Verification items for the finished model (mm, model axes). Face numbers are marked on the shaded views. A direction names the side the tool comes from. Coordinates: 2 decimals unless noted, no trailing zeros. Loops run counter-clockwise (first coordinate to the right, second up) from the corner with the lowest first, then second, coordinate; pieces in that order, holes last. Notation, with made-up numbers: (-24, 17.25) - (-13, 17.25) arc R21 cw to (-13, 44.25) - close; hole circle Ø1 at (88, 42). An arc over 180 degrees is marked (long way). One line per item, written item: value. Start each with the question number.
(1) Draft check along X on the marked faces 6, 7 and 8. Enter one of: +X half, -X half, draft (parallel to the pull), parting line (faces both ways), or undercut.
(2) Set-up check for the marked faces 1, 2, 3, 4 and 5: record each of +Z, -Z, +X, -X, +Y, -Y from which the full face is reachable in a straight line by a thin tool's end or side.
(3) Section check A-A (x = 99). Record the boundary of the cut face in (y, z).
(4) Section check C-C (x = 104). Record the boundary of the cut face in (y, z), plus the area to 3 significant figures.
(5) Gauge pin test, flat ends, axial feed: P1, Ø0.5, axis at y = -1, z = 0.5, coming from the -X side; P2, Ø0.5, axis at x = 108, z = 0.5, coming from the +Y side; P3, Ø2, axis at x = 101, y = -4.5, coming from the -Z side; P4, Ø0.8, axis at y = -0.5, z = 0.5, coming from the +X side. Record the tip position at first contact, or that the pin passes through.
(6) Section check B-B (x = 112.25). Record the boundary of the cut face in (y, z).
(7) Thickness scan on probe 1 along X at (y, z) = (-1, 0.9); probe 2 along X at (y, z) = (-0.75, 1.45); probe 3 along X at (y, z) = (3.25, 1.35). Record the ranges inside material, lowest first. Write a range as [from, to].
```python
from build123d import *

# Parameters (mm, degrees)
BOSS_EXTRUDE1_DEPTH = 1.524


with BuildPart() as part:
    # Sketch1 → Boss-Extrude1 (new body)
    with BuildSketch(Plane.XY):
        with BuildLine():
            Line((106.800157748, 0), (106.800157748, -1.524))
            ThreePointArc((106.800157748, -1.524), (105.191459449, -2.771684776), (103.266120199, -2.110098583))
            ThreePointArc((103.266120199, -2.110098583), (101.457479492, -0.162046547), (100.437603623, 2.292732701))
            Line((100.437603623, 2.292732701), (99.671504405, 2.600209915))
            Line((99.671504405, 2.600209915), (100.220071172, 3.966999231))
            Line((100.220071172, 3.966999231), (98.805734154, 4.534649474))
            Line((98.805734154, 4.534649474), (98.257167386, 3.167860158))
            Line((98.257167386, 3.167860158), (97.491068168, 3.475337373))
            ThreePointArc((97.491068168, 3.475337373), (97.707736418, 2.534285361), (97.993480897, 1.611856983))
            Line((97.993480897, 1.611856983), (99.233794217, 2.047797072))
            Line((99.233794217, 2.047797072), (99.580941947, 0.500608663))
            Line((99.580941947, 0.500608663), (98.60492848, 0.15756357))
            ThreePointArc((98.60492848, 0.15756357), (100.713257844, -2.911730159), (103.603390941, -5.259654218))
            Line((103.603390941, -5.259654218), (104.347526725, -4.013018416))
            Line((104.347526725, -4.013018416), (105.672752741, -4.804065888))
            Line((105.672752741, -4.804065888), (104.974997158, -5.973001868))
            ThreePointArc((104.974997158, -5.973001868), (105.580159309, -6.225365098), (106.197246416, -6.446977219))
            ThreePointArc((106.197246416, -6.446977219), (107.562157749, -7.48677465), (108.927069081, -6.446977219))
            ThreePointArc((108.927069081, -6.446977219), (109.544156188, -6.225365098), (110.14931834, -5.973001868))
            Line((110.14931834, -5.973001868), (109.451562757, -4.804065888))
            Line((109.451562757, -4.804065888), (110.776788773, -4.013018416))
            Line((110.776788773, -4.013018416), (111.520924556, -5.259654218))
            ThreePointArc((111.520924556, -5.259654218), (114.411057653, -2.911730159), (116.519387018, 0.15756357))
            Line((116.519387018, 0.15756357), (115.543373551, 0.500608663))
            Line((115.543373551, 0.500608663), (115.89052128, 2.047797072))
            Line((115.89052128, 2.047797072), (117.130834601, 1.611856983))
            ThreePointArc((117.130834601, 1.611856983), (117.41657908, 2.534285361), (117.63324733, 3.475337373))
            Line((117.63324733, 3.475337373), (116.867148112, 3.167860158))
            Line((116.867148112, 3.167860158), (116.318581344, 4.534649474))
            Line((116.318581344, 4.534649474), (114.904244325, 3.966999231))
            Line((114.904244325, 3.966999231), (115.452811093, 2.600209915))
            Line((115.452811093, 2.600209915), (114.686711874, 2.292732701))
            ThreePointArc((114.686711874, 2.292732701), (113.666836006, -0.162046547), (111.858195299, -2.110098583))
            ThreePointArc((111.858195299, -2.110098583), (109.932856049, -2.771684776), (108.32415775, -1.524))
            Line((108.32415775, -1.524), (108.32415775, 0))
            Line((108.32415775, 0), (106.800157748, 0))
        make_face()
    extrude(amount=BOSS_EXTRUDE1_DEPTH)


solid = part.part
```
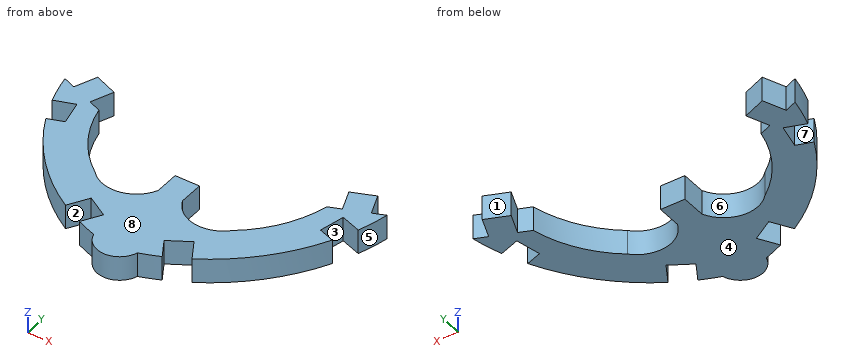
Responses:
1. face 6: undercut
1. face 7: -X half
1. face 8: draft
2. face 1: +Z, -Z, +Y
2. face 2: +Z, -Z, -Y
2. face 3: +Z, -Z
2. face 4: -Z, +X, -X, +Y, -Y
2. face 5: +Z, -Z, +X, -Y
3. outline: (-0.58, 0) - (0.3, 0) - (0.3, 1.52) - (-0.58, 1.52) - close; (1.97, 0) - (4.46, 0) - (4.46, 1.52) - (1.97, 1.52) - close
4. outline: (-4.6, 0) - (-2.63, 0) - (-2.63, 1.52) - (-4.6, 1.52) - close
4. area: 3.00 mm²
5. P1: stops at x = 99.1
5. P2: stops at y = 0
5. P3: stops at z = 0
5. P4: stops at x = 116.39
6. outline: (-4.79, 0) - (-1.79, 0) - (-1.79, 1.52) - (-4.79, 1.52) - close
7. probe 1: x = [99.25, 102.08], [106.8, 108.32], [113.04, 115.87]
7. probe 2: x = [99.1, 101.88], [106.8, 108.32], [113.25, 116.03]
7. probe 3: x = [97.54, 98.05], [98.29, 99.93], [115.19, 116.83], [117.07, 117.59]
